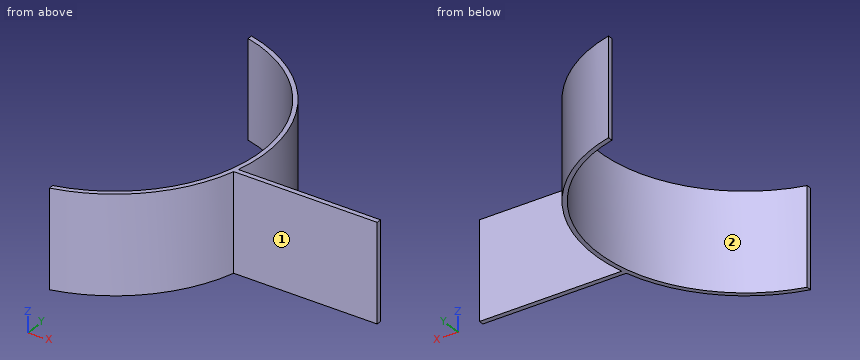
from build123d import *

# Parameters (mm, degrees)
F1_DEPTH = 100


with BuildPart() as f1:
    # F0 (on Top) → F1 (new body)
    with BuildSketch(Plane.XY):
        with BuildLine():
            Line((152.842064, -34.568323), (299.473815, -34.568323))
            Line((299.473815, -34.568323), (299.473815, -29.568323))
            Line((299.473815, -29.568323), (154.109696, -29.568323))
            ThreePointArc((154.109696, -29.568323), (135.118218, 86.86006), (39.976107, 156.604046))
            Line((39.976107, 156.604046), (39.976107, 151.604046))
            ThreePointArc((39.976107, 151.604046), (153.551571, 6.017862), (39.976107, -139.568323))
            Line((39.976107, -139.568323), (39.976107, -144.568323))
            ThreePointArc((39.976107, -144.568323), (111.459598, -105.010963), (152.842064, -34.568323))
        make_face()
    extrude(amount=F1_DEPTH)


solid = f1.part
Can you work these out from the model? Positions are in its coordinate system, mm. Face numbers are marked on the shaded views. Coordinates: 2 decimals unless noted, no trailing zeros. Order: outer loops, then holes, each group sorted by start corner. A loop starts at its lowest first (then second) coordinate and runs counter-clockwise, first axis right, second up. Notation, with made-up numbers: M 9,8.25 L 33,8.25 A21 cw 33,45.25 Z; hole C 52,77.25 d6. An arc over 180 degrees is marked long. Write item = value, one per line.
(1) Suppose I cut it at D-D on y = 112. Please give me the cut outline in (x, z).
Results are:
outline = M 109.74,0 L 115.94,0 L 115.94,100 L 109.74,100 Z
(2) Suppose I cut it at A-A on z = 59. Please give me the cut outline in (x, y).
Results are:
outline = M 39.98,-144.57 A154.77 ccw 152.84,-34.57 L 299.47,-34.57 L 299.47,-29.57 L 154.11,-29.57 A155.8 ccw 39.98,156.6 L 39.98,151.6 A150.1 cw 39.98,-139.57 Z
(3) For pin 1 Ø1.5 at (y, z) = (110.5, 16.5) entering from +X; pin 2 Ø10 at (y, z) = (-38.5, 65) entering from -X; pin 3 Ø2 at (x, z) = (271.5, 15) entering from -Y, each with a flat end and sliding along its axis, tell me the tip position at first contact or that it passes through.
Results are:
pin_1 = 118.01
pin_2 = 145.15
pin_3 = -34.57
(4) Suppose I cut it at B-B on x = 111. Please give me the cut outline in (y, z), plus the area to 3 significant figures.
Results are:
outline = M -105.46,0 L -98.69,0 L -98.69,100 L -105.46,100 Z; M 110.72,0 L 117.04,0 L 117.04,100 L 110.72,100 Z
area = 1,310 mm2
(5) If we mould it in two halves opening along Y, with no side actions, what happens to the marked faces 1 and 2? For each: pulls with the +Y half, pulls with the -Y half, needs draft (parallel to the pull), parting line crosses it, or undercut.
Results are:
face_1 = pulls with the -Y half
face_2 = undercut
(6) I need wall thicknesses on line 1 along Y through (x, z) = (260.5, 4.5); line 2 along Y through (x, z) = (134.5, 63); line 3 along X through (y, z) = (2.5, 67). Which ranges of each line are inside material? Lowest first, please. Write a range as [from, to].
Results are:
line_1 = [-34.57, -29.57]
line_2 = [-76.49, -67.17], [79.2, 87.86]
line_3 = [153.51, 158.06]
(7) Suppose I cut it at C-C on x = 81. Please give me the cut outline in (y, z).
Results are:
outline = M -128.11,0 L -122.5,0 L -122.5,100 L -128.11,100 Z; M 134.53,0 L 139.89,0 L 139.89,100 L 134.53,100 Z
